from build123d import *

# Parameters (mm, degrees)
F0_W     = 25.4
F0_H     = 25.4
F1_DEPTH = 12.7
F2_R     = 6.35
F3_DEPTH = 25.4
F5_DEPTH = 6.3246


with BuildPart() as f1:
    # F0 (on Front) → F1 (new body, symmetric)
    with BuildSketch(Plane.XZ):
        with Locations((12.7, 12.7)):
            Rectangle(F0_W, F0_H)
    extrude(amount=F1_DEPTH, both=True)

    # F2 (on face) → F3 (cut, through all)
    with BuildSketch(Plane.XY.offset(25.4)):
        with Locations((12.7, 0)):
            Circle(F2_R)
    extrude(amount=-F3_DEPTH, mode=Mode.SUBTRACT)

    # F4 (on face) → F5 (cut)
    with BuildSketch(Plane.XZ.offset(12.7)):
        Polygon((15.875, 22.225), (9.525, 22.225), (9.525, 15.875), (3.175, 15.875), (3.175, 9.525), (9.525, 9.525), (9.525, 3.175), (15.875, 3.175), (15.875, 9.525), (22.225, 9.525), (22.225, 15.875), (15.875, 15.875), align=None)
    extrude(amount=-F5_DEPTH, mode=Mode.SUBTRACT)


solid = f1.part
Part model, mm, in its own coordinate system. A direction names the side the tool comes from. Coordinates: 2 decimals unless noted, no trailing zeros. Order: outer loops, then holes, each group sorted by start corner. A loop starts at its lowest first (then second) coordinate and runs counter-clockwise, first axis right, second up. Notation, with made-up numbers: (-36, 61) - (5, 61) arc R32 cw to (5, 100) - close; hole circle Ø7 at (66.5, 82.25). An arc over 180 degrees is marked (long way). Use CSV: the item, a comma, the result in double quotes.
Item 1: Saw through at A-A on x = 12.7. Give the cut face in (y, z) (3 decimals), and give its area (3 significant figures).
Solved:
outline,"(-12.7, 0) - (-6.35, 0) - (-6.35, 25.4) - (-12.7, 25.4) - (-12.7, 22.225) - (-6.375, 22.225) - (-6.375, 3.175) - (-12.7, 3.175) - close; (6.35, 0) - (12.7, 0) - (12.7, 25.4) - (6.35, 25.4) - close"
area,"202 mm²"
Item 2: Probe probe 1 along Z at (x, y) = (8.25, -9.75) (3 decimals); probe 2 along Y at (x, z) = (17.75, 21.5); probe 3 along X at (y, z) = (0.75, 9.5). List the from-to ranges inside material, lowest first.
Solved:
probe 1,"z = 0 to 9.525, 15.875 to 25.4"
probe 2,"y = -12.7 to -3.85, 3.85 to 12.7"
probe 3,"x = 0 to 6.39, 19.01 to 25.4"
Item 3: Saw through at B-B on y = 0. Give the cut face in (x, z), and give its area (3 significant figures).
Solved:
outline,"(0, 0) - (6.35, 0) - (6.35, 25.4) - (0, 25.4) - close; (19.05, 0) - (25.4, 0) - (25.4, 25.4) - (19.05, 25.4) - close"
area,"323 mm²"
Item 4: 3-axis set-ups, long thin cutter, end or side, ignore diameter. For faces 1 (the face through (6.356, 0.279, 12.878)), 2 (the face through (15.875, -10, 6)): which of +Z, -Z, +X, -X, +Y, -Y reach the whole face in a straight line?
Solved:
face 1,"+Z, -Z"
face 2,"-Y"
Item 5: Saw through at C-C on z = 8.25. Give the cut face in (x, y) (3 decimals).
Solved:
outline,"(0, -12.7) - (9.525, -12.7) - (9.525, -6.375) - (15.875, -6.375) - (15.875, -12.7) - (25.4, -12.7) - (25.4, 12.7) - (0, 12.7) - close; hole circle Ø12.7 at (12.7, 0)"
Item 6: Saw through at D-D on x = 4. Give the cut face in (y, z) (3 decimals).
Solved:
outline,"(-12.7, 0) - (12.7, 0) - (12.7, 25.4) - (-12.7, 25.4) - (-12.7, 15.875) - (-6.375, 15.875) - (-6.375, 9.525) - (-12.7, 9.525) - close"
Item 7: Mould opens along X. For faces 3 (the face through (18, -12.7, 7)), 4 (the face through (9.525, -10, 19)), 5 (the face through (0, 0, 13)) say: +X half, -X half, draft (parallel to the pull), parting line (faces both ways), or undercut.
Solved:
face 3,"draft"
face 4,"undercut"
face 5,"-X half"
